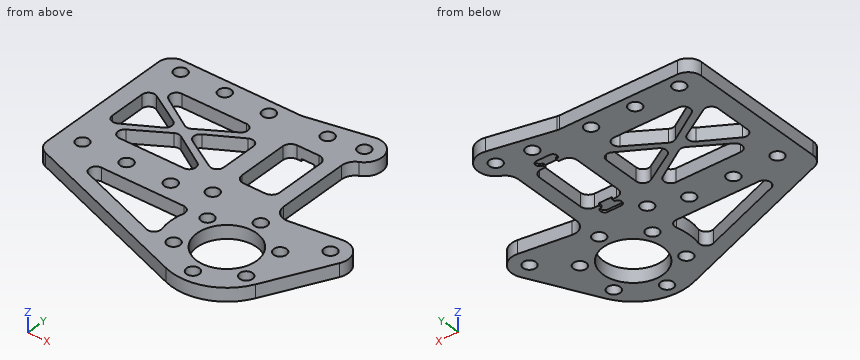
from build123d import *

# Parameters (mm, degrees)
SKETCH_2_R          = 6.75
SKETCH_2_R_2        = 1.45
EXTRUDE_1_DEPTH     = 3
EXTRUDE_START       = -3
SKETCH_4_R          = 1.45
EXTRUDE_2_DEPTH     = 3
SKETCH_5_R          = 1.45
SKETCH_5_W          = 8.5
SKETCH_5_H          = 15
EXTRUDE_3_DEPTH     = 3
SKETCH_7_R          = 1.45
CUT_EXTRUDE_3_DEPTH = 20
FILLET_1_R          = 1.8
FILLET_2_R          = 3
SKETCH_9_R          = 1.45
CUT_EXTRUDE_5_DEPTH = 10.5
FILLET_3_R          = 1.5
SKETCH_10_W         = 3
SKETCH_10_H         = 20
CUT_EXTRUDE_6_DEPTH = 0.5
SKETCH_11_R         = 0.9
CUT_EXTRUDE_7_DEPTH = 0.5


with BuildPart() as part:
    # 草图2 → 凸台-拉伸1 (new body)
    with BuildSketch(Plane.XY):
        with BuildLine():
            Line((-10, -7), (-10, -16.423561614))
            Line((-10, -16.423561614), (30.724748208, -31.24615776))
            ThreePointArc((30.724748208, -31.24615776), (47.310096913, -21.670602221), (35, -7))
            Line((35, -7), (-10, -7))
        make_face()
        with Locations((35, -19.5)):
            Circle(SKETCH_2_R, mode=Mode.SUBTRACT)
        with Locations((15, -10.5)):
            Circle(SKETCH_2_R_2, mode=Mode.SUBTRACT)
        with Locations((5, -10.5)):
            Circle(SKETCH_2_R_2, mode=Mode.SUBTRACT)
        with Locations((-5, -10.5)):
            Circle(SKETCH_2_R_2, mode=Mode.SUBTRACT)
    extrude(amount=EXTRUDE_1_DEPTH)

    # 草图4 → 凸台-拉伸2 (add)
    with BuildSketch(Plane.XY.offset(3).offset(EXTRUDE_START)):
        with BuildLine():
            Line((35, -7), (49.461817276, -5.036370432))
            ThreePointArc((49.461817276, -5.036370432), (53.268884157, -6.694702543), (53.552947171, -10.837543578))
            Line((53.552947171, -10.837543578), (46.102959909, -25.24232368))
            ThreePointArc((46.102959909, -25.24232368), (45.677758332, -13.00111725), (35, -7))
        make_face()
        with Locations((50, -9)):
            Circle(SKETCH_4_R, mode=Mode.SUBTRACT)
    extrude(amount=EXTRUDE_2_DEPTH)

    # 草图5 → 凸台-拉伸3 (add)
    with BuildSketch(Plane(origin=(0, 0, 0), x_dir=(-1, 0, 0), z_dir=(0, 0, -1))):
        with BuildLine():
            Line((-35, -7), (-35, 15))
            ThreePointArc((-35, 15), (-38.979463437, 19.404809528), (-34.194537642, 22.918064623))
            Line((-34.194537642, 22.918064623), (-20, 20))
            Line((-20, 20), (10, 20))
            Line((10, 20), (10, -7))
            Line((10, -7), (-35, -7))
        make_face()
        with Locations((-35, 19)):
            Circle(SKETCH_5_R, mode=Mode.SUBTRACT)
        with Locations((-27.5, 5)):
            Rectangle(SKETCH_5_W, SKETCH_5_H, mode=Mode.SUBTRACT)
    extrude(amount=-EXTRUDE_3_DEPTH)

    # 草图7 → 切除-拉伸3 (cut)
    with BuildSketch(Plane.XY.offset(3)):
        with Locations((27.5, 18)):
            Circle(SKETCH_7_R)
        with Locations((-5, 17)):
            Circle(SKETCH_7_R)
        with Locations((5, 17)):
            Circle(SKETCH_7_R)
        with Locations((15, 17)):
            Circle(SKETCH_7_R)
        with Locations((22.5, -8)):
            Circle(SKETCH_7_R)
    extrude(amount=-CUT_EXTRUDE_3_DEPTH, mode=Mode.SUBTRACT)

    # 圆角1
    fillet_1_edges = [part.edges().sort_by_distance(p)[0] for p in [
        (31.75, 12.5, 1.5),
        (23.25, 12.5, 1.5),
        (23.25, -2.5, 1.5),
        (31.75, -2.5, 1.5),
    ]]
    fillet(fillet_1_edges, radius=FILLET_1_R)

    # 圆角2
    fillet_2_edges = [part.edges().sort_by_distance(p)[0] for p in [
        (35, 15, 1.5),
        (20, 20, 1.5),
        (-10, 20, 1.5),
        (35, -7, 1.5),
        (-10, -16.423561614, 1.5),
    ]]
    fillet(fillet_2_edges, radius=FILLET_2_R)

    # 草图9 → 切除-拉伸5 (cut)
    with BuildSketch(Plane(origin=(0, 0, 0), x_dir=(-1, 0, 0), z_dir=(0, 0, -1))):
        with Locations((-26.772758664, -14.75)):
            Circle(SKETCH_9_R)
        with Locations((-26.772758664, -24.25)):
            Circle(SKETCH_9_R)
        with Locations((-35, -29)):
            Circle(SKETCH_9_R)
        with Locations((-43.227241336, -24.25)):
            Circle(SKETCH_9_R)
        with Locations((-43.227241336, -14.75)):
            Circle(SKETCH_9_R)
        with Locations((-35, -10)):
            Circle(SKETCH_9_R)
        Polygon((-6.625, 4.25), (-19.25, 12), (6, 12), align=None)
        Polygon((-7.625, 3.25), (-19.25, 10), (-19.25, -3.5), align=None)
        Polygon((6, 10), (6, -3.5), (-5.625, 3.25), align=None)
        Polygon((-19.25, -5.5), (6, -5.5), (-6.625, 2.25), align=None)
        with BuildLine():
            Line((-23.271295894, -14.5), (6, -14.5))
            Line((6, -14.5), (-23.639402612, -25.287860312))
            ThreePointArc((-23.639402612, -25.287860312), (-22.257416141, -19.934806402), (-23.271295894, -14.5))
        make_face()
    extrude(amount=-CUT_EXTRUDE_5_DEPTH, mode=Mode.SUBTRACT)

    # 圆角3
    fillet_3_edges = [part.edges().sort_by_distance(p)[0] for p in [
        (5.625, 3.25, 1.5),
        (-6, 10, 1.5),
        (-6, -3.5, 1.5),
        (19.25, -5.5, 1.5),
        (6.625, 2.25, 1.5),
        (-6, -5.5, 1.5),
        (23.639402612, -25.287860312, 1.5),
        (23.271295894, -14.5, 1.5),
        (-6, -14.5, 1.5),
        (7.625, 3.25, 1.5),
        (19.25, -3.5, 1.5),
        (19.25, 10, 1.5),
        (-6, 12, 1.5),
        (6.625, 4.25, 1.5),
        (19.25, 12, 1.5),
    ]]
    fillet(fillet_3_edges, radius=FILLET_3_R)

    # 草图10 → 切除-拉伸6 (cut)
    with BuildSketch(Plane(origin=(0, 0, 0), x_dir=(-1, 0, 0), z_dir=(0, 0, -1))):
        with Locations((-27.5, 5)):
            Rectangle(SKETCH_10_W, SKETCH_10_H)
    extrude(amount=-CUT_EXTRUDE_6_DEPTH, mode=Mode.SUBTRACT)

    # 草图11 → 切除-拉伸7 (cut)
    with BuildSketch(Plane(origin=(0, 0, 0), x_dir=(-1, 0, 0), z_dir=(0, 0, -1))):
        with Locations((-29, 14.1)):
            Circle(SKETCH_11_R)
        with Locations((-26, 14.1)):
            Circle(SKETCH_11_R)
        with Locations((-29, -4.1)):
            Circle(SKETCH_11_R)
        with Locations((-26, -4.1)):
            Circle(SKETCH_11_R)
    extrude(amount=-CUT_EXTRUDE_7_DEPTH, mode=Mode.SUBTRACT)


solid = part.part
Can you work these out from the model? Positions are in its coordinate system, mm. Round coordinates to 2 decimals unless told otherwise and drop trailing zeros. Write each loop counter-clockwise with the first axis right and the second up, starting at its lowest first coordinate (ties: lowest second). Pieces come first, ordered by that corner, then holes. Notation, with made-up numbers: M -32.75,-28.5 L 12.25,-28.5 A21 ccw 12.25,-12.5 Z; hole C 57,21 d1. An arc over 180 degrees is marked long. Use a Markdown table: item, result.
Item 1: I want a section at B-B (y = -29). List the corners of the cut face in (x, z) for me, and give its area (3 significant figures).
Found:
| item | result |
|---|---|
| outline | M 24.55,0 L 33.55,0 L 33.55,3 L 24.55,3 Z; M 36.45,0 L 43.12,0 L 43.12,3 L 36.45,3 Z |
| area | 47.0 mm2 |
Item 2: I want a section at D-D (y = 5.5). List the corners of the cut face in (x, z) for me, and give its area (3 significant figures).
Found:
| item | result |
|---|---|
| outline | M -10,0 L -6,0 L -6,3 L -10,3 Z; M 1.75,0 L 4.59,0 L 4.59,3 L 1.75,3 Z; M 8.66,0 L 11.5,0 L 11.5,3 L 8.66,3 Z; M 19.25,0 L 23.25,0 L 23.25,3 L 19.25,3 Z; M 31.75,0 L 35,0 L 35,3 L 31.75,3 Z |
| area | 50.8 mm2 |
Item 3: For pin 1 Ø1.5 at (x, z) = (16, 1.5) entering from -Y; pin 2 Ø0.9 at (x, z) = (27, 1) entering from -Y; pin 3 Ø1.5 at (x, z) = (9, 2) entering from +Y, each with a flat end and sliding along its axis, tell me the tip position at first contact or that it passes through.
Found:
| item | result |
|---|---|
| pin 1 | stops at y = -26.16 |
| pin 2 | stops at y = -30.05 |
| pin 3 | stops at y = 20 |
Item 4: I want a section at A-A (x = 43). List the corners of the cut face in (y, z) for me.
Found:
| item | result |
|---|---|
| outline | M -29.1,0 L -25.68,0 L -25.68,3 L -29.1,3 Z; M -22.82,0 L -16.18,0 L -16.18,3 L -22.82,3 Z; M -13.32,0 L -5.91,0 L -5.91,3 L -13.32,3 Z |
Item 5: If I drill on line 1 along Y through (x, z) = (27.5, 1.35); line 2 along X through (y, z) = (0, 1.25); line 3 along X through (y, z) = (7, 1.15), over which ranges is the centre line in solid material (lowest first)? Write a range as [from, to].
Found:
| item | result |
|---|---|
| line 1 | y = [-30.07, -25.5], [-23, -16], [-13.5, -2.5], [12.5, 16.55], [19.45, 21.54] |
| line 2 | x = [-10, -6], [0.03, 2.96], [10.29, 13.22], [19.25, 23.25], [31.75, 35] |
| line 3 | x = [-10, -6], [-0.83, 2.15], [11.1, 14.08], [19.25, 23.25], [31.75, 35] |
Item 6: I want a section at C-C (x = 27.5). List the corners of the cut face in (y, z) for me, and give its area (3 significant figures).
Found:
| item | result |
|---|---|
| outline | M -30.07,0 L -25.5,0 L -25.5,3 L -30.07,3 Z; M -23,0 L -16,0 L -16,3 L -23,3 Z; M -13.5,0 L -5,0 L -5,0.5 L -2.5,0.5 L -2.5,3 L -13.5,3 Z; M 12.5,0.5 L 15,0.5 L 15,0 L 16.55,0 L 16.55,3 L 12.5,3 Z; M 19.45,0 L 21.54,0 L 21.54,3 L 19.45,3 Z |
| area | 83.6 mm2 |
